```python
from build123d import *

# Parameters (mm, degrees)
BASE_FLANGE1_DEPTH  = 31.75
SKETCH6_R           = 4.3688
CUT_EXTRUDE1_DEPTH  = 337.385219094
SKETCH7_R           = 2.4511
SKETCH7_R_2         = 9.525
CUT_EXTRUDE2_DEPTH  = 337.385219094
SKETCH8_R           = 4.3688
BOSS_EXTRUDE1_DEPTH = 3.175
FILLET1_R           = 6.35
FILLET2_R           = 3.175


# Sheet-metal steps are written as plain solids
with BuildPart() as part:
    # Sketch1 → Base-Flange1 (new body)
    with BuildSketch(Plane(origin=(0, 0, 0), x_dir=(0, 0, -1), z_dir=(1, 0, 0))):
        with BuildLine():
            Line((31.75, 0), (6.35, 0))
            ThreePointArc((6.35, 0), (1.859871939, -1.859871939), (0, -6.35))
            Line((0, -6.35), (0, -333.375))
            Line((0, -333.375), (3.175, -333.375))
            Line((3.175, -333.375), (3.175, -6.35))
            ThreePointArc((3.175, -6.35), (4.10493597, -4.10493597), (6.35, -3.175))
            Line((6.35, -3.175), (31.75, -3.175))
            Line((31.75, -3.175), (31.75, 0))
        make_face()
    extrude(amount=BASE_FLANGE1_DEPTH)

    # Sketch6 → Cut-Extrude1 (cut, through all)
    with BuildSketch(Plane(origin=(0, 0, 0), x_dir=(1, 0, 0), z_dir=(0, 1, 0))):
        with Locations(Location((19.05, 22.225, 0), (0, 0, 270))):
            Circle(SKETCH6_R)
    extrude(amount=-CUT_EXTRUDE1_DEPTH, mode=Mode.SUBTRACT)

    # Sketch7 → Cut-Extrude2 (cut, through all)
    with BuildSketch(Plane.XY):
        with Locations((19.05, -79.375)):
            Circle(SKETCH7_R)
        with Locations((19.05, -320.675)):
            Circle(SKETCH7_R)
        with Locations((15.875, -38.1)):
            Circle(SKETCH7_R_2)
    extrude(amount=-CUT_EXTRUDE2_DEPTH, mode=Mode.SUBTRACT)

    # Sketch8 → Boss-Extrude1 (add)
    with BuildSketch(Plane.XY):
        Polygon((-107.95, -180.975), (-107.95, -114.3), (0, -6.35), (0, -180.975), align=None)
        with Locations((-88.9, -117.475)):
            Circle(SKETCH8_R, mode=Mode.SUBTRACT)
        with Locations((-19.05, -117.475)):
            Circle(SKETCH8_R, mode=Mode.SUBTRACT)
        with Locations((-88.9, -168.275)):
            Circle(SKETCH8_R, mode=Mode.SUBTRACT)
        with Locations((-19.05, -168.275)):
            Circle(SKETCH8_R, mode=Mode.SUBTRACT)
    extrude(amount=-BOSS_EXTRUDE1_DEPTH)

    # Fillet1
    fillet1_edges = [part.edges().sort_by_distance(p)[0] for p in [
        (0, -180.975, -1.5875),
    ]]
    fillet(fillet1_edges, radius=FILLET1_R)

    # Fillet2
    fillet2_edges = [part.edges().sort_by_distance(p)[0] for p in [
        (0, -6.35, -1.5875),
        (31.75, -1.5875, -31.75),
        (-107.95, -180.975, -1.5875),
        (-107.95, -114.3, -1.5875),
        (0, -1.5875, -31.75),
        (31.75, -333.375, -1.5875),
        (0, -333.375, -1.5875),
    ]]
    fillet(fillet2_edges, radius=FILLET2_R)


solid = part.part
```
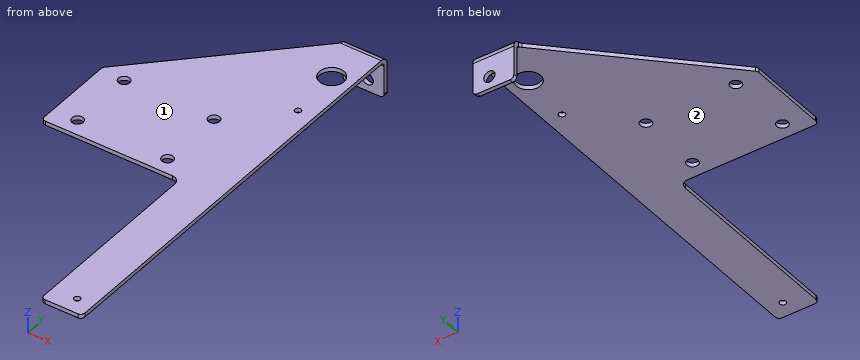
Source: CAD feature listing. Evaluate the final solid. Frame: model axes, mm. Face numbers are marked on the shaded views. A direction names the side the tool comes from. Give positions to 0.01 mm unless a question says otherwise; leave off trailing zeros. Write each loop counter-clockwise with the first axis right and the second up, starting at its lowest first coordinate (ties: lowest second). Pieces come first, ordered by that corner, then holes.
1. Section query C-C (z = -22). Return the cut outline in (x, y) (3 decimals), then the cut area to 3 significant figures.
2. Section query B-B (x = -19.05). Return the cut outline in (y, z) (3 decimals), then the cut area to 3 significant figures.
3. Material intervals for line 1 along Y through (x, z) = (-88.9, -1.15) (3 decimals); line 2 along Z through (x, y) = (-17.5, -41) (3 decimals); line 3 along Y through (x, z) = (19.05, -2.05) (3 decimals), sorted ascending.
4. Access query for the marked faces 1 and 2. Directions: +Z, -Z, +X, -X, +Y, -Y. A direction counts if a zero-diameter tool reaches every point of the face in a straight line with its end or side. Return the directions, or none.
5. First-contact query: pin 1 (8 mm diameter, centred on x = -19.05, y = -168.275, fed in from -Z); pin 2 (10 mm diameter, centred on x = -19.05, y = -117.475, fed in from -Z) (3 decimals); pin 3 (5.5 mm diameter, centred on y = -3.5, z = -19.5, fed in from -X); pin 4 (10 mm diameter, centred on x = 19.05, z = -22.225, fed in from -Y) (3 decimals). Flat tips, straight axial feed; report the tip coordinate or a pass-through.
6. Section query D-D (x = -88.9). Return the cut outline in (y, z) (3 decimals), then the cut area to 3 significant figures.
7. Section query A-A (y = -38.1). Return the cut outline in (x, z) (3 decimals).
Output values:
1. outline: (0, -3.175) - (14.687, -3.175) - (14.687, 0) - (0, 0) - close; (23.413, -3.175) - (31.75, -3.175) - (31.75, 0) - (23.413, 0) - close
1. area: 73.1 mm2
2. outline: (-180.975, -3.175) - (-172.644, -3.175) - (-172.644, 0) - (-180.975, 0) - close; (-163.906, -3.175) - (-121.844, -3.175) - (-121.844, 0) - (-163.906, 0) - close; (-113.106, -3.175) - (-25.4, -3.175) - (-25.4, 0) - (-113.106, 0) - close
2. area: 438 mm2
3. line 1: y = -180.975 to -172.644, -163.906 to -121.844, -113.106 to -95.25
3. line 2: z = -3.175 to 0
3. line 3: y = -333.375 to -323.126, -318.224 to -81.826, -76.924 to -47.08, -29.12 to -1.677
4. face 1: +Z, +X, -X, +Y, -Y
4. face 2: -Z, +X, -X, -Y
5. pin 1: passes through
5. pin 2: stops at z = -3.175
5. pin 3: stops at x = 0
5. pin 4: stops at y = -3.175
6. outline: (-180.975, -3.175) - (-172.644, -3.175) - (-172.644, 0) - (-180.975, 0) - close; (-163.906, -3.175) - (-121.844, -3.175) - (-121.844, 0) - (-163.906, 0) - close; (-113.106, -3.175) - (-95.25, -3.175) - (-95.25, 0) - (-113.106, 0) - close
6. area: 217 mm2
7. outline: (-31.75, -3.175) - (6.35, -3.175) - (6.35, 0) - (-31.75, 0) - close; (25.4, -3.175) - (31.75, -3.175) - (31.75, 0) - (25.4, 0) - close
